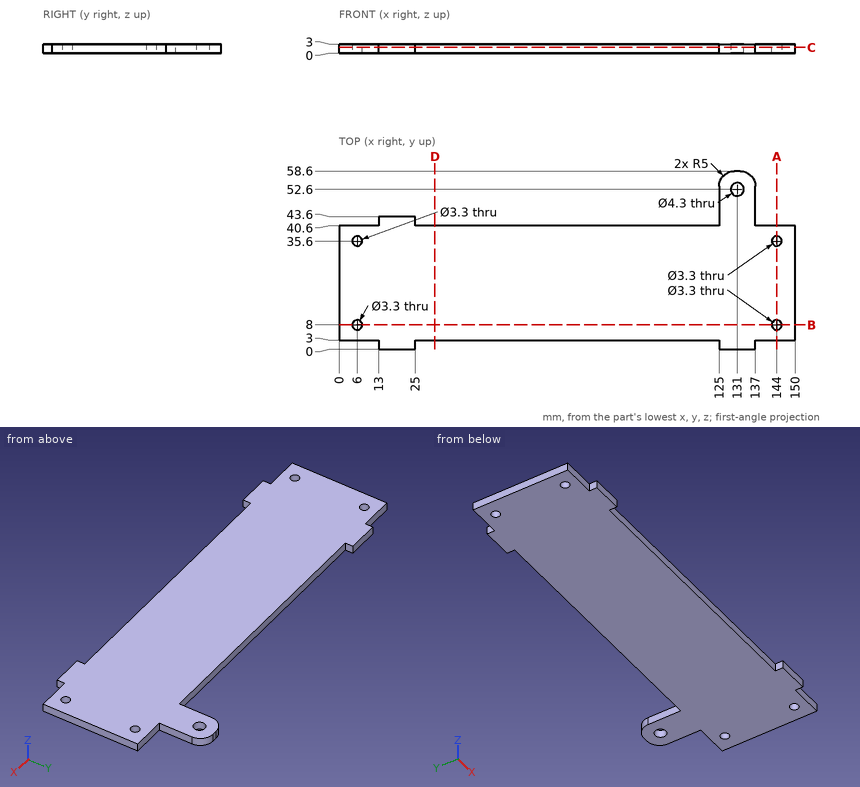
Print and shaded views of the part. All mm, measured from the part's lowest x, y and z. Coordinates: 2 decimals unless noted, no trailing zeros. Order: outer loops, then holes, each group sorted by start corner. A loop starts at its lowest first (then second) coordinate and runs counter-clockwise, first axis right, second up. Notation, with made-up numbers: M -26,21 L 11,21 A22 ccw 11,30 Z; hole C 59,28 d4. An arc over 180 degrees is marked long. Answer as CSV lines item,"result".
1) Cut at D-D (x = 31.5). List the corners of the cut face in (y, z).
Verdict:
outline,"M 3,0 L 40.6,0 L 40.6,3 L 3,3 Z"
2) Cut at C-C (z = 1.9). List the corners of the cut face in (x, y).
Verdict:
outline,"M 0,3 L 13,3 L 13,0 L 25,0 L 25,3 L 125,3 L 125,0 L 137,0 L 137,3 L 150,3 L 150,40.6 L 137,40.6 L 137,53.6 A5 ccw 132,58.6 L 130,58.6 A5 ccw 125,53.6 L 125,40.6 L 25,40.6 L 25,43.6 L 13,43.6 L 13,40.6 L 0,40.6 Z; hole C 6,8 d3.3; hole C 6,35.6 d3.3; hole C 131,52.6 d4.3; hole C 144,8 d3.3; hole C 144,35.6 d3.3"
3) Drill centre lines: L1, parallel to Y at x = 6, z = 1; L2, parallel to Y at x = 32, z = 1.45; L3, parallel to Y at x = 130, z = 0.85. Where is each one in solid material? Low to high. Write a range as from..to.
Verdict:
L1,"3..6.35, 9.65..33.95, 37.25..40.6"
L2,"3..40.6"
L3,"0..50.7, 54.5..58.6"
4) Cut at A-A (x = 144). List the corners of the cut face in (y, z), then the cut area to 3 significant figures.
Verdict:
outline,"M 3,0 L 6.35,0 L 6.35,3 L 3,3 Z; M 9.65,0 L 33.95,0 L 33.95,3 L 9.65,3 Z; M 37.25,0 L 40.6,0 L 40.6,3 L 37.25,3 Z"
area,"93.0 mm2"
5) Flat gauge pins, fed straight in: P1, Ø0.9, axis at x = 21, z = 2, coming from the +Y side; P2, Ø1, axis at x = 62.5, z = 2, coming from the +Y side; P3, Ø1.5, axis at x = 61.5, z = 1, coming from the -Y side. Where does each tip first touch, or does it go through?
Verdict:
P1,"y = 43.6"
P2,"y = 40.6"
P3,"y = 3"
6) Cut at B-B (y = 8). List the corners of the cut face in (x, z), then the cut area to 3 significant figures.
Verdict:
outline,"M 0,0 L 4.35,0 L 4.35,3 L 0,3 Z; M 7.65,0 L 142.35,0 L 142.35,3 L 7.65,3 Z; M 145.65,0 L 150,0 L 150,3 L 145.65,3 Z"
area,"430 mm2"
